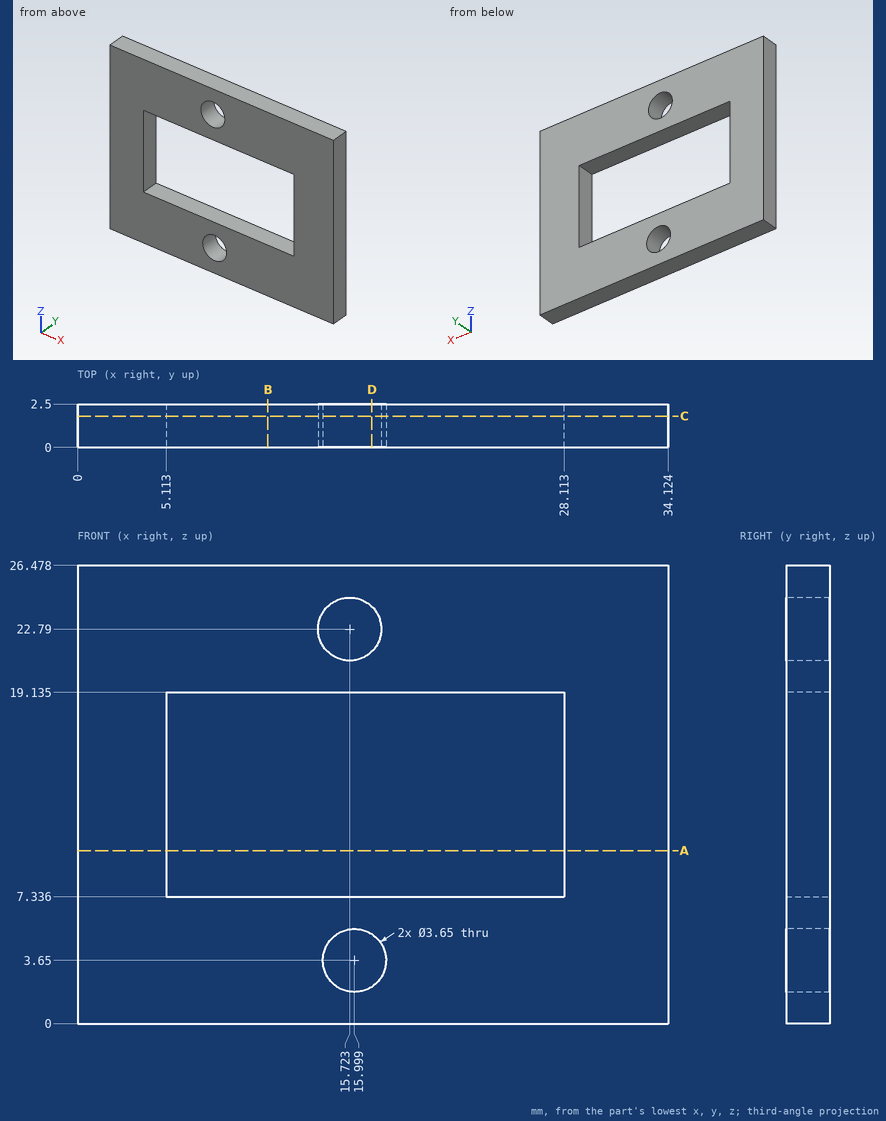
Here's the drawing with two shaded views (mm, measured from the low corner). I have some questions. Coordinates: 2 decimals unless noted, no trailing zeros. Write each loop counter-clockwise with the first axis right and the second up, starting at its lowest first coordinate (ties: lowest second). Pieces come first, ordered by that corner, then holes. Notation, with made-up numbers: (14.5, -20) - (53.5, -20) arc R16 ccw to (53.5, -7) - close; hole circle Ø11 at (-31.5, -26). An arc over 180 degrees is marked (long way). Return JSON: item names as keys, results as strings.
Q1. If we section it at C-C (y = 1.8): Count the separate pieces of the cut face and the enclosed holes in it, then the cut area to 3 significant figures.
Computed values:
{"separate pieces": "1", "enclosed holes": "3", "area": "611 mm2"}
Q2. If we section it at A-A (z = 10): Please give me the cut outline in (x, y) (1 decimal).
Computed values:
{"outline": "(0, 0) - (5.1, 0) - (5.1, 2.5) - (0, 2.5) - close; (28.1, 0) - (34.1, 0) - (34.1, 2.5) - (28.1, 2.5) - close"}
Q3. If we section it at D-D (x = 17): Please give me the cut outline in (y, z) (1 decimal).
Computed values:
{"outline": "(0, 0) - (2.5, 0) - (2.5, 2.1) - (0, 2.1) - close; (0, 5.2) - (2.5, 5.2) - (2.5, 7.3) - (0, 7.3) - close; (0, 19.1) - (2.5, 19.1) - (2.5, 21.5) - (0, 21.5) - close; (0, 24.1) - (2.5, 24.1) - (2.5, 26.5) - (0, 26.5) - close"}
Q4. Please list where these lines run through material, in increasing order: L1, parallel to X at y = 0.9, z = 16.5 (1 decimal); L2, parallel to Z at x = 23.5, y = 1.2 (1 decimal); L3, parallel to X at y = 0.45, z = 21.25 (1 decimal). Write a range as from..to.
Computed values:
{"L1": "x = 0..5.1, 28.1..34.1", "L2": "z = 0..7.3, 19.1..26.5", "L3": "x = 0..14.7, 16.7..34.1"}
Q5. If we section it at B-B (x = 11): Please give me the cut outline in (y, z) (1 decimal), then the cut area to 3 significant figures.
Computed values:
{"outline": "(0, 0) - (2.5, 0) - (2.5, 7.3) - (0, 7.3) - close; (0, 19.1) - (2.5, 19.1) - (2.5, 26.5) - (0, 26.5) - close", "area": "36.7 mm2"}
Q6. I'm going to push a flat-ended pin straight in: pin 1 Ø4 at (x, z) = (15.72, 22.79) entering from +Y. Where does the tip first touch, or does it pass through?
Computed values:
{"pin 1": "stops at y = 2.5"}
